Job drawing, mm, ordinate dimensions from the low corner. One solid piece. A direction names the side the tool comes from. Round coordinates to 2 decimals unless told otherwise and drop trailing zeros. Order: outer loops, then holes, each group sorted by start corner. A loop starts at its lowest first (then second) coordinate and runs counter-clockwise, first axis right, second up. Notation, with made-up numbers: (-8.75, -18) -> (49.25, -18) arc R34 ccw to (49.25, 12) -> close; hole circle Ø11 at (-28, 67). An arc over 180 degrees is marked (long way). Write item = value, one per line.
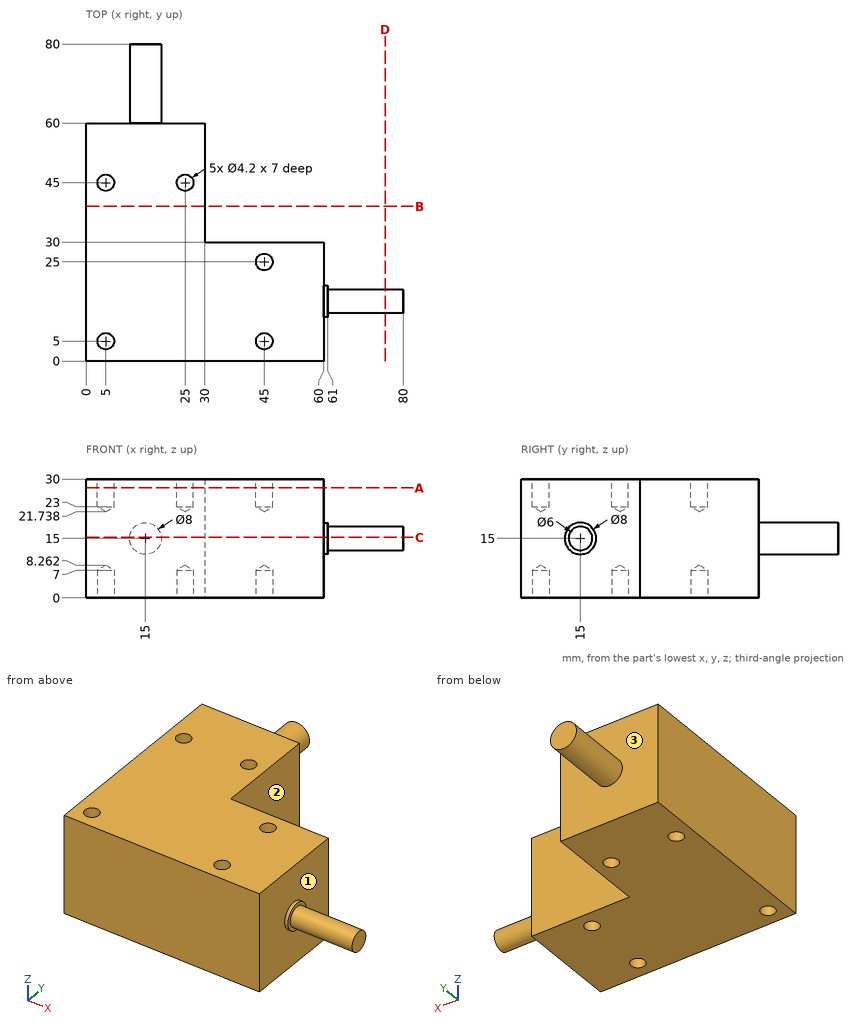
Q1. Cut at A-A, the plane z = 27.75. List the corners of the cut face in (x, y), and give its area (3 significant figures).
Check values:
outline = (0, 0) -> (60, 0) -> (60, 30) -> (30, 30) -> (30, 60) -> (0, 60) -> close; hole circle Ø4.2 at (5, 5); hole circle Ø4.2 at (5, 45); hole circle Ø4.2 at (25, 45); hole circle Ø4.2 at (45, 5); hole circle Ø4.2 at (45, 25)
area = 2,630 mm²
Q2. Flat gauge pins, fed straight in: pin 1 (3 mm diameter, centred on x = 20.5, z = 10.5, fed in from +Y); pin 2 (4 mm diameter, centred on x = 5, y = 5, fed in from +Z); pin 3 (2.5 mm diameter, centred on x = 45, y = 25, fed in from +Z). Where does each tip first touch, or does it go through?
Check values:
pin_1 = 60
pin_2 = 22.94
pin_3 = 22.49
Q3. Cut at B-B, the plane y = 39. List the corners of the cut face in (x, z).
Check values:
outline = (0, 0) -> (30, 0) -> (30, 30) -> (0, 30) -> close
Q4. Probe probe 1 along X at (y, z) = (5, 3.5); probe 2 along X at (y, z) = (45, 27). List the from-to ranges inside material, lowest first.
Check values:
probe_1 = 0 to 2.9, 7.1 to 42.9, 47.1 to 60
probe_2 = 0 to 2.9, 7.1 to 22.9, 27.1 to 30
Q5. Cut at C-C, the plane z = 15.25. List the corners of the cut face in (x, y).
Check values:
outline = (0, 0) -> (60, 0) -> (60, 11.01) -> (61, 11.01) -> (61, 12.01) -> (80, 12.01) -> (80, 17.99) -> (61, 17.99) -> (61, 18.99) -> (60, 18.99) -> (60, 30) -> (30, 30) -> (30, 60) -> (18.99, 60) -> (18.99, 80) -> (11.01, 80) -> (11.01, 60) -> (0, 60) -> close
Q6. Cut at D-D, the plane x = 75.5. List the corners of the cut face in (y, z).
Check values:
outline = circle Ø6 at (15, 15)
Q7. Which spindle directions (+Z, -Z, +X, -X, +Y, -Y) get a long thin tool onto all of the face, cutting with end or side? Do the marked faces 1, 2 and 3. Say none if no direction does.
Check values:
face_1 = +X
face_2 = +Z, -Z, +X, +Y
face_3 = +Y
